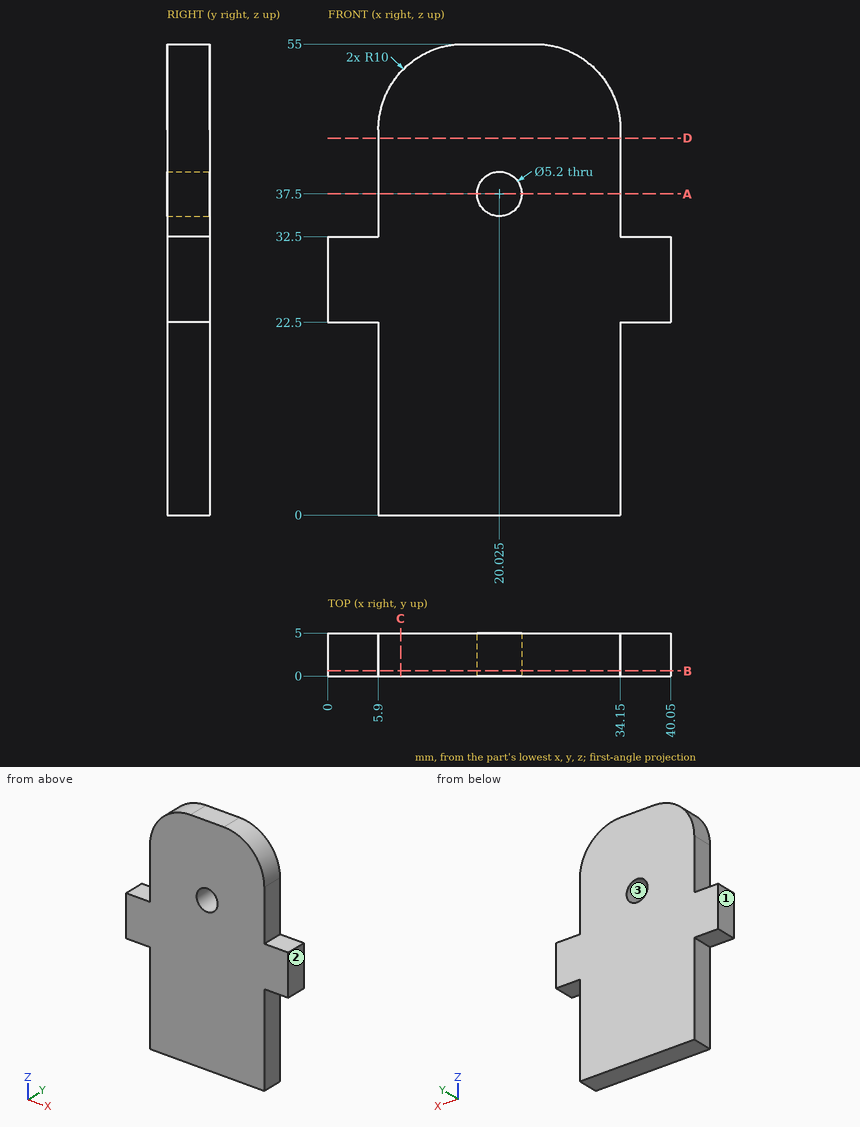
Study the drawing (mm; zero at the part's minimum x, y, z) and answer. Round coordinates to 2 decimals unless told otherwise and drop trailing zeros. Write each loop counter-clockwise with the first axis right and the second up, starting at its lowest first coordinate (ties: lowest second). Pieces come first, ordered by that corner, then holes.
1) A cutting plane is placed at A-A on z = 37.5. Determine the outline of the cut face in (x, y) (3 decimals), and give its area (3 significant figures).
2) A cutting plane is placed at C-C on x = 8.5. Determine the outline of the cut face in (y, z), and give its area (3 significant figures).
3) Consider probe 1 along X at (y, z) = (3.15, 37.5) (3 decimals); probe 2 along X at (y, z) = (1.6, 17); probe 3 along Z at (x, y) = (4, 2.9). Determine where each line is inside the solid, lowest interval first.
4) Determine the mould class of the marked faces 1, 2 and 3 for opening direction X: pulls with the +X half, pulls with the -X half, needs draft (parallel to the pull), parting line crosses it, or undercut.
5) A cutting plane is placed at B-B on y = 0.6. Determine the outline of the cut face in (x, z) (3 decimals).
6) A cutting plane is placed at D-D on z = 44. Determine the outline of the cut face in (x, y).
7) Flat-ended cylindrical pins translate along their axes: P1, Ø12, axis at x = 16, z = 33.5, coming from the -Y side; P2, Ø2.5, axis at x = 1.5, y = 1.5, coming from the -Z side; P3, Ø1.5, axis at x = 38, y = 3, coming from the +Z side; P4, Ø2.5, axis at y = 3, z = 12, coming from the -X side. Find the tip coordinate at first contact, or state that the pin passes through.
Entries:
1. outline: (5.9, 0) - (17.425, 0) - (17.425, 5) - (5.9, 5) - close; (22.625, 0) - (34.15, 0) - (34.15, 5) - (22.625, 5) - close
1. area: 115 mm2
2. outline: (0, 0) - (5, 0) - (5, 51.73) - (0, 51.73) - close
2. area: 259 mm2
3. probe 1: x = 5.9 to 17.425, 22.625 to 34.15
3. probe 2: x = 5.9 to 34.15
3. probe 3: z = 22.5 to 32.5
4. face 1: pulls with the -X half
4. face 2: pulls with the +X half
4. face 3: undercut
5. outline: (0, 22.5) - (5.9, 22.5) - (5.9, 0) - (34.15, 0) - (34.15, 22.5) - (40.05, 22.5) - (40.05, 32.5) - (34.15, 32.5) - (34.15, 45) arc R10 ccw to (24.15, 55) - (15.9, 55) arc R10 ccw to (5.9, 45) - (5.9, 32.5) - (0, 32.5) - close; hole circle Ø5.2 at (20.025, 37.5)
6. outline: (5.9, 0) - (34.15, 0) - (34.15, 5) - (5.9, 5) - close
7. P1: stops at y = 0
7. P2: stops at z = 22.5
7. P3: stops at z = 32.5
7. P4: stops at x = 5.9
